Read the model definition and answer for the solid it produces. Units are mm, in the model's axes. Coordinates: 2 decimals unless noted, no trailing zeros. Loops run counter-clockwise (first coordinate to the right, second up) from the corner with the lowest first, then second, coordinate; pieces in that order, holes last. Notation, with made-up numbers: (74.5, 13) -> (104.5, 13) arc R19 ccw to (104.5, 35) -> close; hole circle Ø2 at (61.25, 30.25). An arc over 180 degrees is marked (long way). Answer in a Markdown table with one row per item.
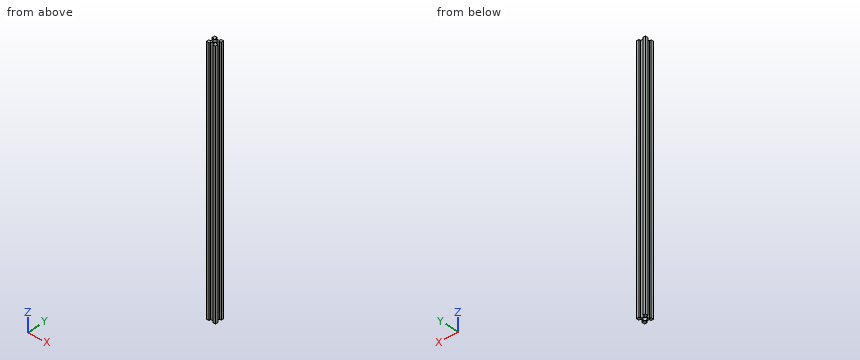
```python
from build123d import *

# Parameters (mm, degrees)
F1_DEPTH = 71.12


with BuildPart() as f1:
    # F0 (on Top) → F1 (new body)
    with BuildSketch(Plane.XY):
        Polygon((0, 0.773533), (0, 0), (0.769862, 0), (0.769862, 0.507953), (1.781597, 0.507953), (1.781597, 0), (2.54, 0), (2.54, 0.773533), (2.03453, 0.773533), (2.03453, 1.785268), (2.54, 1.785268), (2.54, 2.54), (1.781597, 2.54), (1.781597, 2.038202), (0.757215, 2.038202), (0.757215, 2.54), (0, 2.54), (0, 1.785268), (0.516928, 1.785268), (0.516928, 1.27), (0.516928, 0.773533), align=None)
        with BuildLine():
            ThreePointArc((1.780828, 1.27), (1.263083, 0.752255), (0.745338, 1.27))
            ThreePointArc((0.745338, 1.27), (1.263083, 1.787745), (1.780828, 1.27))
        make_face(mode=Mode.SUBTRACT)
    extrude(amount=F1_DEPTH)


solid = f1.part
```
1. A cutting plane is placed at A-A on z = 43. Give the vertices of the cut face in (x, y).
A:
| item | result |
|---|---|
| outline | (0, 0) -> (0.77, 0) -> (0.77, 0.51) -> (1.78, 0.51) -> (1.78, 0) -> (2.54, 0) -> (2.54, 0.77) -> (2.03, 0.77) -> (2.03, 1.79) -> (2.54, 1.79) -> (2.54, 2.54) -> (1.78, 2.54) -> (1.78, 2.04) -> (0.76, 2.04) -> (0.76, 2.54) -> (0, 2.54) -> (0, 1.79) -> (0.52, 1.79) -> (0.52, 0.77) -> (0, 0.77) -> close; hole circle Ø1.04 at (1.26, 1.27) |
2. Find the intervals of material crossed by probe 1 along X at (y, z) = (1.25, 11.5); probe 2 along Y at (x, z) = (1.25, 6.5); probe 3 along X at (y, z) = (2.25, 37.5), in increasing order.
A:
| item | result |
|---|---|
| probe 1 | x = 0.52 to 0.75, 1.78 to 2.03 |
| probe 2 | y = 0.51 to 0.75, 1.79 to 2.04 |
| probe 3 | x = 0 to 0.76, 1.78 to 2.54 |
3. Given pin 1 Ø1.1 at (y, z) = (1, 42.5) entering from +X; pin 2 Ø0.5 at (x, z) = (1.5, 24.5) entering from -Y, each flat-ended and moving along its own axis, determine where each tip first touches the part or whether it passes through.
A:
| item | result |
|---|---|
| pin 1 | stops at x = 2.54 |
| pin 2 | stops at y = 0.51 |
4. A cutting plane is placed at B-B on y = 1.27. Give the vertices of the cut face in (x, z), and give its area (3 significant figures).
A:
| item | result |
|---|---|
| outline | (0.52, 0) -> (0.75, 0) -> (0.75, 71.12) -> (0.52, 71.12) -> close; (1.78, 0) -> (2.03, 0) -> (2.03, 71.12) -> (1.78, 71.12) -> close |
| area | 34.3 mm2 |
